from build123d import *

# Parameters (mm, degrees)
F0_R     = 3.05
F1_DEPTH = 10


with BuildPart() as f1:
    # F0 (on Front) → F1 (new body)
    with BuildSketch(Plane.XZ):
        with BuildLine():
            ThreePointArc((5.987557, -1.959377), (6.221399, -0.992066), (6.3, 0))
            ThreePointArc((6.3, 0), (6.25371, 0.762306), (6.115521, 1.513409))
            ThreePointArc((6.115521, 1.513409), (5.905269, 2.194948), (5.619331, 2.848354))
            ThreePointArc((5.619331, 2.848354), (4.615787, 4.287716), (3.254184, 5.394468))
            ThreePointArc((3.254184, 5.394468), (2.623594, 5.727718), (1.959377, 5.987557))
            ThreePointArc((1.959377, 5.987557), (0.231982, 6.295727), (-1.513409, 6.115521))
            ThreePointArc((-1.513409, 6.115521), (-2.194948, 5.905269), (-2.848354, 5.619331))
            ThreePointArc((-2.848354, 5.619331), (-4.287716, 4.615787), (-5.394468, 3.254184))
            ThreePointArc((-5.394468, 3.254184), (-5.727718, 2.623594), (-5.987557, 1.959377))
            ThreePointArc((-5.987557, 1.959377), (-6.295727, 0.231982), (-6.115521, -1.513409))
            ThreePointArc((-6.115521, -1.513409), (-5.905269, -2.194948), (-5.619331, -2.848354))
            ThreePointArc((-5.619331, -2.848354), (-4.615787, -4.287716), (-3.254184, -5.394468))
            ThreePointArc((-3.254184, -5.394468), (-2.623594, -5.727718), (-1.959377, -5.987557))
            ThreePointArc((-1.959377, -5.987557), (-0.231982, -6.295727), (1.513409, -6.115521))
            ThreePointArc((1.513409, -6.115521), (2.194948, -5.905269), (2.848354, -5.619331))
            ThreePointArc((2.848354, -5.619331), (4.287716, -4.615787), (5.394468, -3.254184))
            ThreePointArc((5.394468, -3.254184), (5.727718, -2.623594), (5.987557, -1.959377))
        make_face()
        Circle(F0_R, mode=Mode.SUBTRACT)
        with BuildLine():
            ThreePointArc((6.115521, 1.513409), (6.25371, 0.762306), (6.3, 0))
            ThreePointArc((6.3, 0), (6.221399, -0.992066), (5.987557, -1.959377))
            ThreePointArc((5.987557, -1.959377), (6.194917, -1.692674), (6.524551, -1.618716))
            Line((6.524551, -1.618716), (8.996032, -1.926502))
            ThreePointArc((8.996032, -1.926502), (7.594846, -0.279851), (9.113417, 1.259215))
            Line((9.113417, 1.259215), (6.625987, 1.134152))
            ThreePointArc((6.625987, 1.134152), (6.30269, 1.232169), (6.115521, 1.513409))
        make_face()
        with BuildLine():
            ThreePointArc((3.254184, 5.394468), (4.615787, 4.287716), (5.619331, 2.848354))
            ThreePointArc((5.619331, 2.848354), (5.577369, 3.183566), (5.758159, 3.468949))
            Line((5.758159, 3.468949), (7.723398, 4.998913))
            ThreePointArc((7.723398, 4.998913), (5.568251, 5.172483), (5.55376, 7.334559))
            Line((5.55376, 7.334559), (3.883314, 5.487247))
            ThreePointArc((3.883314, 5.487247), (3.585399, 5.32795), (3.254184, 5.394468))
        make_face()
        with BuildLine():
            ThreePointArc((5.487247, -3.883314), (5.32795, -3.585399), (5.394468, -3.254184))
            ThreePointArc((5.394468, -3.254184), (4.287716, -4.615787), (2.848354, -5.619331))
            ThreePointArc((2.848354, -5.619331), (3.183566, -5.577369), (3.468949, -5.758159))
            Line((3.468949, -5.758159), (4.998913, -7.723398))
            ThreePointArc((4.998913, -7.723398), (5.172483, -5.568251), (7.334559, -5.55376))
            Line((7.334559, -5.55376), (5.487247, -3.883314))
        make_face()
        with BuildLine():
            ThreePointArc((10.793761, -0.338767), (10.29636, 0.820662), (9.113417, 1.259215))
            ThreePointArc((9.113417, 1.259215), (7.594846, -0.279851), (8.996032, -1.926502))
            ThreePointArc((8.996032, -1.926502), (10.252919, -1.538009), (10.793761, -0.338767))
        make_face()
        with BuildLine():
            ThreePointArc((-1.513409, 6.115521), (0.231982, 6.295727), (1.959377, 5.987557))
            ThreePointArc((1.959377, 5.987557), (1.692674, 6.194917), (1.618716, 6.524551))
            Line((1.618716, 6.524551), (1.926502, 8.996032))
            ThreePointArc((1.926502, 8.996032), (0.279851, 7.594846), (-1.259215, 9.113417))
            Line((-1.259215, 9.113417), (-1.134152, 6.625987))
            ThreePointArc((-1.134152, 6.625987), (-1.232169, 6.30269), (-1.513409, 6.115521))
        make_face()
        with BuildLine():
            ThreePointArc((5.55376, 7.334559), (5.568251, 5.172483), (7.723398, 4.998913))
            ThreePointArc((7.723398, 4.998913), (8.17798, 5.558793), (8.340515, 6.261426))
            ThreePointArc((8.340515, 6.261426), (7.31549, 7.754545), (5.55376, 7.334559))
        make_face()
        with BuildLine():
            ThreePointArc((1.134152, -6.625987), (1.232169, -6.30269), (1.513409, -6.115521))
            ThreePointArc((1.513409, -6.115521), (-0.231982, -6.295727), (-1.959377, -5.987557))
            ThreePointArc((-1.959377, -5.987557), (-1.692674, -6.194917), (-1.618716, -6.524551))
            Line((-1.618716, -6.524551), (-1.926502, -8.996032))
            ThreePointArc((-1.926502, -8.996032), (-0.279851, -7.594846), (1.259215, -9.113417))
            Line((1.259215, -9.113417), (1.134152, -6.625987))
        make_face()
        with BuildLine():
            ThreePointArc((7.861426, -6.740515), (7.723789, -6.091289), (7.334559, -5.55376))
            ThreePointArc((7.334559, -5.55376), (5.172483, -5.568251), (4.998913, -7.723398))
            ThreePointArc((4.998913, -7.723398), (6.781031, -8.253793), (7.861426, -6.740515))
        make_face()
        with BuildLine():
            ThreePointArc((-5.394468, 3.254184), (-4.287716, 4.615787), (-2.848354, 5.619331))
            ThreePointArc((-2.848354, 5.619331), (-3.183566, 5.577369), (-3.468949, 5.758159))
            Line((-3.468949, 5.758159), (-4.998913, 7.723398))
            ThreePointArc((-4.998913, 7.723398), (-4.748148, 7.260119), (-4.661426, 6.740515))
            ThreePointArc((-4.661426, 6.740515), (-5.612201, 5.278152), (-7.334559, 5.55376))
            Line((-7.334559, 5.55376), (-5.487247, 3.883314))
            ThreePointArc((-5.487247, 3.883314), (-5.32795, 3.585399), (-5.394468, 3.254184))
        make_face()
        with BuildLine():
            ThreePointArc((-1.259215, 9.113417), (0.279851, 7.594846), (1.926502, 8.996032))
            ThreePointArc((1.926502, 8.996032), (1.935698, 9.094706), (1.938767, 9.193761))
            ThreePointArc((1.938767, 9.193761), (0.298582, 10.793256), (-1.259215, 9.113417))
        make_face()
        with BuildLine():
            ThreePointArc((-3.883314, -5.487247), (-3.585399, -5.32795), (-3.254184, -5.394468))
            ThreePointArc((-3.254184, -5.394468), (-4.615787, -4.287716), (-5.619331, -2.848354))
            ThreePointArc((-5.619331, -2.848354), (-5.577369, -3.183566), (-5.758159, -3.468949))
            Line((-5.758159, -3.468949), (-7.723398, -4.998913))
            ThreePointArc((-7.723398, -4.998913), (-6.037881, -4.823961), (-5.140515, -6.261426))
            ThreePointArc((-5.140515, -6.261426), (-5.247396, -6.836401), (-5.55376, -7.334559))
            Line((-5.55376, -7.334559), (-3.883314, -5.487247))
        make_face()
        with BuildLine():
            ThreePointArc((1.261233, -9.193761), (1.260729, -9.153576), (1.259215, -9.113417))
            ThreePointArc((1.259215, -9.113417), (-0.279851, -7.594846), (-1.926502, -8.996032))
            ThreePointArc((-1.926502, -8.996032), (-0.437821, -10.790692), (1.261233, -9.193761))
        make_face()
        with BuildLine():
            ThreePointArc((-6.115521, -1.513409), (-6.295727, 0.231982), (-5.987557, 1.959377))
            ThreePointArc((-5.987557, 1.959377), (-6.194917, 1.692674), (-6.524551, 1.618716))
            Line((-6.524551, 1.618716), (-8.996032, 1.926502))
            ThreePointArc((-8.996032, 1.926502), (-7.994518, 1.397925), (-7.593761, 0.338767))
            ThreePointArc((-7.593761, 0.338767), (-8.034332, -0.763833), (-9.113417, -1.259215))
            Line((-9.113417, -1.259215), (-6.625987, -1.134152))
            ThreePointArc((-6.625987, -1.134152), (-6.30269, -1.232169), (-6.115521, -1.513409))
        make_face()
        with BuildLine():
            ThreePointArc((-4.661426, 6.740515), (-4.748148, 7.260119), (-4.998913, 7.723398))
            ThreePointArc((-4.998913, 7.723398), (-7.35037, 7.912778), (-7.334559, 5.55376))
            ThreePointArc((-7.334559, 5.55376), (-5.612201, 5.278152), (-4.661426, 6.740515))
        make_face()
        with BuildLine():
            ThreePointArc((-7.723398, -4.998913), (-7.912778, -7.35037), (-5.55376, -7.334559))
            ThreePointArc((-5.55376, -7.334559), (-5.247396, -6.836401), (-5.140515, -6.261426))
            ThreePointArc((-5.140515, -6.261426), (-6.037881, -4.823961), (-7.723398, -4.998913))
        make_face()
        with BuildLine():
            ThreePointArc((-7.593761, 0.338767), (-7.994518, 1.397925), (-8.996032, 1.926502))
            ThreePointArc((-8.996032, 1.926502), (-10.792676, 0.397683), (-9.113417, -1.259215))
            ThreePointArc((-9.113417, -1.259215), (-8.034332, -0.763833), (-7.593761, 0.338767))
        make_face()
    extrude(amount=F1_DEPTH)


solid = f1.part
Can you work these out from the model? Positions are in its coordinate system, mm. A direction names the side the tool comes from. Give positions to 0.01 mm unless a question says otherwise; leave off trailing zeros. Order: outer loops, then holes, each group sorted by start corner. A loop starts at its lowest first (then second) coordinate and runs counter-clockwise, first axis right, second up. Notation, with made-up numbers: M -11.75,-33 L 14.25,-33 A31 ccw 14.25,1 Z; hole C 74,55 d11. An arc over 180 degrees is marked long. Use a Markdown table: item, result. Add a question column.
Item 1: Will these pins go through, and if not, where does the flat tip stop? pin 1 (3 mm diameter, centred on x = -8, y = -6, fed in from +Z); pin 2 (2 mm diameter, centred on y = -8.5, z = 3, fed in from -X); pin 3 (1 mm diameter, centred on x = -8.5, y = -6.5, fed in from -Z); pin 4 (5.5 mm diameter, centred on x = 0, z = 0, fed in from +Y).
Item 2: For faces 1 (the cylindrical face through (5.909, -4.93, 2.186)), 2 (the cylindrical face through (-5.909, -4.93, -2.186)), 3 (the flat face through (4.73, -4.93, 6.424)), 4 (the flat face through (7.74, -4.93, -1.77)), 5 (the flat face through (2, 0, 3)), which set-ups out of +Z, -Z, +X, -X, +Y, -Y let a thin tool reach every point of the face, with its end or its side?
Item 3: Suppose I cut it at B-B (z = 0). List the corners of the cut face in (x, y) for me, then the cut area to 3 significant figures.
Item 4: We'd pull the mould along Z, two halves only. Please class faces 6 (the cylindrical face through (2.633, -4.93, 5.724)), 7 (the flat face through (-4.73, -4.93, -6.424)), 8 (the flat face through (-6.424, -4.93, 4.73)): +Z half, -Z half, draft (parallel to the pull), parting line (faces both ways), or undercut.
Item 5: If I drill on L1, parallel to Z at x = -6.5, y = -0.5; L2, parallel to X at y = -5.5, z = -7.25; L3, parallel to X at y = -1.25, z = -7.5 (3 decimals), over which ranges is the centre line in solid material (lowest first)? Write a range as [from, to].
Item 6: Suppose I cut it at A-A (x = -0.5). List the corners of the cut face in (y, z) for me.
Answer sheet:
| question | item | result |
|---|---|---|
| 1 | pin 1 | stops at z = 8.32 |
| 1 | pin 2 | stops at x = -5.97 |
| 1 | pin 3 | stops at z = -7.25 |
| 1 | pin 4 | passes through |
| 2 | face 1 | +X, +Y, -Y |
| 2 | face 2 | -X, +Y, -Y |
| 2 | face 3 | +Z, +Y, -Y |
| 2 | face 4 | +Y, -Y |
| 2 | face 5 | +Z, -Z, +X, -X, +Y |
| 3 | outline | M -10.76,-10 L -3.05,-10 L -3.05,0 L -10.76,0 Z; M 3.05,-10 L 10.76,-10 L 10.76,0 L 3.05,0 Z |
| 3 | area | 154 mm² |
| 4 | face 6 | +Z half |
| 4 | face 7 | -Z half |
| 4 | face 8 | undercut |
| 5 | L1 | z = [-7.84, -4.05], [-1.14, 1.62], [4.8, 8.32] |
| 5 | L2 | x = [-8, -5.48], [-1.71, 1.17], [4.63, 7.78] |
| 5 | L3 | x = [-7.753, -5.728], [-1.74, 1.178], [4.825, 7.67] |
| 6 | outline | M -10,-10.79 L 0,-10.79 L 0,-3.01 L -10,-3.01 Z; M -10,3.01 L 0,3.01 L 0,10.56 L -10,10.56 Z |
